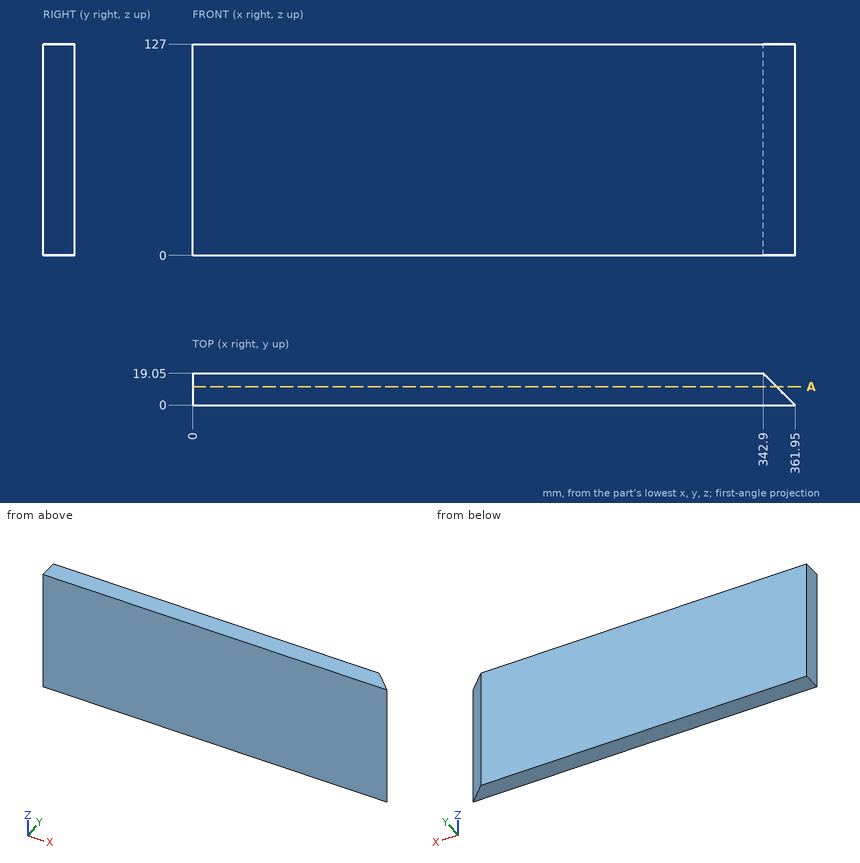
Here's the drawing with two shaded views (mm, measured from the low corner). I have some questions. Coordinates: 2 decimals unless noted, no trailing zeros. Order: outer loops, then holes, each group sorted by start corner. A loop starts at its lowest first (then second) coordinate and runs counter-clockwise, first axis right, second up.
Item 1: For P1, Ø4, axis at y = 14, z = 108.5, coming from the +X side, with a flat end and sliding along its axis, tell me the tip position at first contact or that it passes through.
Result sheet:
P1: stops at x = 349.95
Item 2: If we section it at A-A on y = 11: List the corners of the cut face in (x, z) for me, plus the area to 3 significant figures.
Result sheet:
outline: (0, 0) - (350.95, 0) - (350.95, 127) - (0, 127) - close
area: 44,600 mm2
Item 3: I need wall thicknesses on line 1 (X direction, y = 4.5, z = 25); line 2 (X direction, y = 15, z = 90). Which ranges of each line are inside material? Lowest first, please.
Result sheet:
line 1: x = 0 to 357.45
line 2: x = 0 to 346.95
